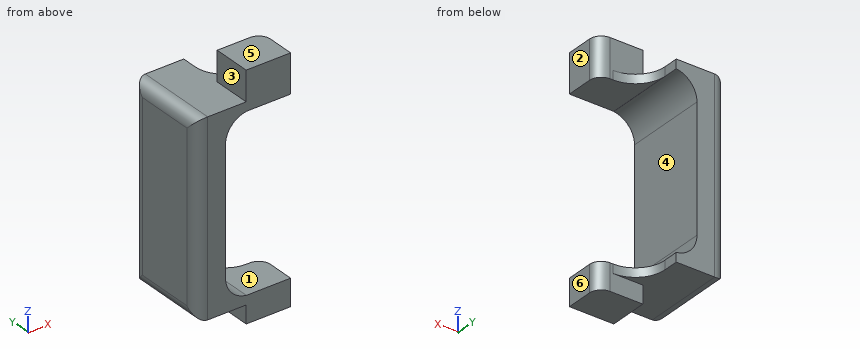
Autodesk Inventor part; units mm, degrees
ref_plane "YZ Plane" through (0, 0, 0) normal (1, 0, 0) x (0, 1, 0)
ref_plane "XZ Plane" through (0, 0, 0) normal (0, 1, 0) x (-1, 0, 0)
ref_plane "XY Plane" through (0, 0, 0) normal (0, 0, 1) x (1, 0, 0)
sketch "Sketch1" plane through (0, 0, 0) normal (0, 1, 0) x (-1, 0, 0)
  line L0 (0.85, 3.2) -> (-0.85, 3.2)
  line L1 (-0.85, 3.2) -> (-0.85, -3.2)
  line L2 (-0.85, -3.2) -> (0.85, -3.2)
  line L3 (0.85, -3.2) -> (0.85, 3.2)
  line L4 (0.85, 3.2) -> (-0.85, -3.2) construction
  line L5 (-0.85, 3.2) -> (0.85, -3.2) construction
  line L6 (-0.85, -1.3) -> (-2.35, -1.3) construction
  line L7 (-2.35, -1.3) -> (-2.35, -3.4525)
  line L8 (-0.85, -3.2) -> (-0.85, -1.3)
  line L9 (-2.35, -3.4525) -> (-2.35, -3.8)
  line L10 (-2.35, -3.8) -> (-0.85, -3.8)
  line L11 (-0.85, -3.8) -> (-0.85, -3.2)
  line L12 (-2.35, -2.9) -> (-0.85, -2.9)
  line L13 (0, 0) -> (-4.1965, 0) construction
  line L14 (-2.35, 1.3) -> (-2.35, 3.4525)
  line L15 (-2.35, 2.9) -> (-0.85, 2.9)
  line L16 (-0.85, 2.9) -> (-2.35, 2.9)
  line L17 (-2.35, 2.9) -> (-2.35, 4.2)
  line L18 (-2.35, 4.2) -> (-0.85, 4.2)
  line L19 (-0.85, 4.2) -> (-0.85, 2.9)
  line L20 (-0.85, 2.9) -> (-0.15, 2.9)
  line L21 (-0.15, 2.9) -> (-0.15, -2.9)
  line L22 (-0.15, -2.9) -> (-0.85, -2.9)
  line L23 (-0.85, -2.9) -> (-0.85, 2.9)
  point P0 (-0.85, 2.9)
  point P1 (-0.85, -2.9)
  point P2 (-2.35, 3.4525)
  point P3 (-0.85, 2.9)
  point P4 (-0.85, -2.9)
  dimension "d0" = 1.3
  dimension "d2" = 1.7
  dimension "d3" = 1.5
  dimension "d5" = 1.9
  dimension "d7" = 2.9
  dimension "d13" = 1
  dimension "d14" = 2.5
  dimension "d18" = 0.7
extrude "Extrusion1" add sketch "Sketch1" along normal blind 2.8 contours L3 L2 L1 L22 L21 L20 L0 | L1 L15 L14 L17 L18 L19 | L11 L10 L9 L7 L12 L1
sketch "Sketch2" plane through (0, 0, 0) normal (0, 0, 1) x (1, 0, 0)
  line L0 (0.85, 2.8) -> (2.35, 2.8)
  line L1 (2.35, 2.8) -> (2.35, 1.3)
  line L2 (2.35, 1.3) -> (0.85, 1.3)
  line L3 (0.85, 1.3) -> (0.85, 2.8)
  line L4 (2.35, 0) -> (2.35, 2.8)
  line L5 (0.85, 0) -> (0.85, 2.8)
  line L6 (0.85, 2.8) -> (2.35, 2.8)
  dimension "d15" = 1.5
extrude "Extrusion2" cut sketch "Sketch2" along normal through all both and the other way through all
fillet "Fillet1" radius 0.8 2 edges at (0.15, 1.4, -2.9) (0.15, 1.4, 2.9)
fillet "Fillet1" radius 1 2 edges at (0.85, 1.3, 3.05) (0.85, 1.3, -3.05)
fillet "Fillet1" radius 0.4 2 edges at (2.35, 1.3, 3.55) (2.35, 1.3, -3.35)
fillet "Fillet1" radius 0.4 4 edges at (-0.85, 2.8, 0) (-0.85, 0, 0) (-0.85, 1.4, -3.2) (-0.85, 1.4, 3.2)
equation "\"button_height\" = 1.3"
properties part number "Button"
Here's how the part is built. I have some questions about the finished solid (model axes, mm). Face numbers are marked on the shaded views. A direction names the side the tool comes from. Give positions to 0.01 mm unless a question says otherwise; leave off trailing zeros. Write each loop counter-clockwise with the first axis right and the second up, starting at its lowest first coordinate (ties: lowest second). Pieces come first, ordered by that corner, then holes. Notation, with made-up numbers: (83.5, 7.5) -> (117.5, 7.5) arc R35 ccw to (117.5, 40.5) -> close; hole circle Ø4 at (37, 74.5). An arc over 180 degrees is marked (long way). Use one line per item in the form item = value. Start each with the question number.
1. Imagine slicing it at C-C on z = 1.25. List the corners of the cut face in (x, y) for me.
2. If I drill on L1, parallel to Z at x = 1.05, y = 1; L2, parallel to X at y = 2.3, z = -1.5; L3, parallel to Z at x = 0.35, y = 2.15, over which ranges is the centre line in solid material (lowest first)?
3. Will these pins go through, and if not, where does the flat tip stop? pin 1 Ø0.9 at (x, z) = (1.5, 3.5) entering from +Y; pin 2 Ø0.7 at (x, y) = (1, 2) entering from +Z; pin 3 Ø0.8 at (y, z) = (1.5, 1) entering from +X.
4. Imagine slicing it at A-A on x = 2.1. List the corners of the cut face in (y, z) for me.
5. On a 3-axis mill with a long thin cutter (end or side, diameter ignored), from which of +Z, -Z, +X, -X, +Y, -Y can I reach the whole of each face in a straight line? I mean the marked faces 1, 2 and 3. Say none if no direction works.
6. Thinking about a two-plate mould opening in Z: for the marked faces 4, 5 and 6, which applies, +Z half, -Z half, draft (parallel to the pull), parting line (faces both ways), or undercut?
Entries:
q1.outline = (-0.85, 0.4) arc R0.4 ccw to (-0.45, 0) -> (0.15, 0) -> (0.15, 2.8) -> (-0.45, 2.8) arc R0.4 ccw to (-0.85, 2.4) -> close
q2.L1 = -3.8 to -2.9, 2.9 to 4.2
q2.L2 = -0.85 to 0.15
q2.L3 = -3.2 to -2.63, 2.63 to 3.2
q3.pin_1 = 1.57
q3.pin_2 = 3.2
q3.pin_3 = 0.15
q4.outline = (0, -3.8) -> (1.27, -3.8) -> (1.27, -2.9) -> (0, -2.9) -> close; (0, 2.9) -> (1.27, 2.9) -> (1.27, 4.2) -> (0, 4.2) -> close
q5.face_1 = +X, +Y, -Y
q5.face_2 = +Z, -Z, +X, +Y, -Y
q5.face_3 = +Z, -X, +Y, -Y
q6.face_4 = undercut
q6.face_5 = +Z half
q6.face_6 = draft
